Can you work these out from the model? Positions are in its coordinate system, mm. Face numbers are marked on the shaded views. Give positions to 0.01 mm unless a question says otherwise; leave off trailing zeros. Write each loop counter-clockwise with the first axis right and the second up, starting at its lowest first coordinate (ties: lowest second). Pieces come first, ordered by that corner, then holes. Notation, with made-up numbers: (20, -8) -> (51, -8) arc R17 cw to (51, 3) -> close; hole circle Ø11 at (-34, 0.25). An arc over 180 degrees is marked (long way). Answer as CSV lines item,"result". Start each with the question number.
1. If we section it at A-A on z = 0: Write out the boundary of the cut face in (x, y).
2. I need wall thicknesses on line 1 (Z direction, x = 10.5, y = 0); line 2 (Y direction, x = 14, z = 8); line 3 (Z direction, x = 7, y = -8). Which ranges of each line are inside material? Lowest first, please. Write a range as [from, to].
3. If we mould it in two halves opening along Z, with no side actions, what happens to the marked faces 1, 2, 3 and 4? For each: pulls with the +Z half, pulls with the -Z half, needs draft (parallel to the pull), parting line crosses it, or undercut.
4. If we section it at B-B on x = 12.75: Write out the boundary of the cut face in (y, z).
5. I'm going to push flat-ended pins straight in: P1, Ø2, axis at y = -7, z = 12.5, coming from the -X side; P2, Ø1.4, axis at y = 7.5, z = 16.5, coming from the +X side; P3, Ø1, axis at x = 13.5, z = 14.5, coming from the +Y side. Where does each tip first touch, or does it pass through?
```python
from build123d import *

# Parameters (mm, degrees)
F0_R     = 19.848958
F0_R_2   = 11.303
F1_DEPTH = 17.78
F2_R     = 7.62
F3_W     = 5.119225
F3_H     = 1.897266
F3_W_2   = 1.970694
F3_H_2   = 4.695322
F3_W_3   = 2.363822
F3_H_3   = 3.009573
F4_DEPTH = 2.54


with BuildPart() as f1:
    # F0 (on Right) → F1 (new body)
    with BuildSketch(Plane.YZ):
        Circle(F0_R)
        Circle(F0_R_2, mode=Mode.SUBTRACT)
    extrude(amount=F1_DEPTH)

    # F2
    f2_edges = [f1.edges().sort_by_distance(p)[0] for p in [
        (17.78, -19.848958, 0),
        (0, -19.848958, 0),
    ]]
    fillet(f2_edges, radius=F2_R)

    # F3 (on Right) → F4 (join)
    with BuildSketch(Plane.YZ):
        Polygon((-16.004974, 2.860423), (-9.045522, 11.621134), (-11.280753, 12.795233), (-17.947224, 4.403334), align=None)
        Polygon((-7.344878, 16.480749), (-8.859969, 16.480749), (-5.829786, 13.28801), (-5.829786, 15.35471), align=None)
        Polygon((-0.795809, 17.064454), (-2.434773, 17.146636), (-2.434773, 13.698089), (0, 13.698089), align=None)
        with Locations((5.589543, 16.248173)):
            Rectangle(F3_W, F3_H)
        Polygon((15.545471, 10.081242), (11.165203, 11.949784), (14.310407, 8.834369), align=None)
        Polygon((15.304292, 6.423779), (13.562527, 6.725411), (13.562527, 2.356187), (15.901389, 2.356187), align=None)
        with Locations((14.825182, -3.328288)):
            Rectangle(F3_W_2, F3_H_2)
        Polygon((8.990117, -10.330278), (8.990117, -13.34158), (12.587023, -11.835929), align=None)
        Polygon((0, -12.875467), (0, -15.095817), (5.354564, -17.308898), (6.13836, -15.412497), align=None)
        Polygon((-2.445628, -13.634987), (-12.557364, -8.420914), (-4.788246, -16.027622), align=None)
        with Locations((-14.094844, -4.16113)):
            Rectangle(F3_W_3, F3_H_3)
    extrude(amount=F4_DEPTH)


solid = f1.part
```
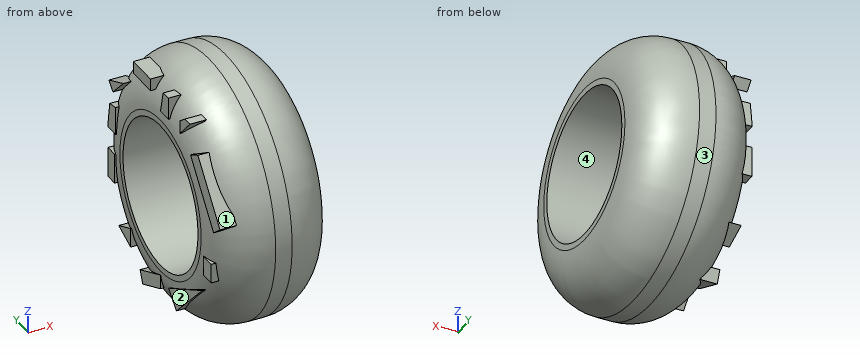
Computed values:
1,outline,"(0, -12.23) arc R7.62 ccw to (7.62, -19.85) -> (10.16, -19.85) arc R7.62 ccw to (17.78, -12.23) -> (17.78, -11.3) -> (0, -11.3) -> close; (0, 11.3) -> (17.78, 11.3) -> (17.78, 12.23) arc R7.62 ccw to (10.16, 19.85) -> (7.62, 19.85) arc R7.62 ccw to (0, 12.23) -> close"
2,line 1,"z = [-19.84, -11.3], [11.3, 19.84]"
2,line 2,"y = [-17.02, -7.98], [7.98, 17.02]"
2,line 3,"z = [-18.14, -7.98], [7.98, 18.14]"
3,face 1,"pulls with the +Z half"
3,face 2,"needs draft"
3,face 3,"parting line crosses it"
3,face 4,"undercut"
4,outline,"circle Ø38.79 at (0, 0); hole circle Ø22.61 at (0, 0)"
5,P1,"stops at x = 0.08"
5,P2,"stops at x = 15.73"
5,P3,"stops at y = 13.06"
